```python
from build123d import *

# Parameters (mm, degrees)
SKETCH1_W                = 254
SKETCH1_H                = 508
BOSS_EXTRUDE1_DEPTH      = 203.2
FILLET1_RADIUS           = 101.6
FILLET1_LENGTH           = 254
BOSS_EXTRUDE2_DEPTH      = 25.4
BOSS_EXTRUDE2_DEPTH_BACK = 279.4
SKETCH2_R                = 12.7
CUT_EXTRUDE1_DEPTH       = 195.834
CUT_EXTRUDE1_DEPTH_BACK  = 440.182
SKETCH4_R                = 12.7


with BuildPart() as part:
    # Sketch1 → Boss-Extrude1 (new body)
    with BuildSketch(Plane.XY):
        with Locations((127, 254)):
            Rectangle(SKETCH1_W, SKETCH1_H)
    extrude(amount=BOSS_EXTRUDE1_DEPTH)

    # Fillet1: full round fillet: the end face becomes a half cylinder, R = half its width
    fillet1_face = Plane((127, 0, 101.6), x_dir=(1, 0, 0), z_dir=(0, -1, 0))  # on the end face: x along it, z out of the body
    fillet1_slab = fillet1_face.offset(-FILLET1_RADIUS / 2) * Box(FILLET1_LENGTH, 2 * FILLET1_RADIUS, FILLET1_RADIUS, mode=Mode.PRIVATE)  # the body's end, R deep
    fillet1_round = Plane((127, 101.6, 101.6), x_dir=(0, -1, 0), z_dir=(1, 0, 0)) * Cylinder(FILLET1_RADIUS, FILLET1_LENGTH, mode=Mode.PRIVATE)  # its axis R under the face
    add(fillet1_slab - fillet1_round, mode=Mode.SUBTRACT)

    # Sketch2 → Boss-Extrude2 (add, two sides: drawn at the far end of the back side and taken through both)
    with BuildSketch(Plane(origin=(254, 0, 0), x_dir=(0, 0, -1), z_dir=(1, 0, 0)).offset(-BOSS_EXTRUDE2_DEPTH_BACK)):
        with Locations((-101.6, 25.4)):
            Circle(SKETCH2_R)
    extrude(amount=BOSS_EXTRUDE2_DEPTH + BOSS_EXTRUDE2_DEPTH_BACK)

    # Sketch4 → Cut-Extrude1 (cut, two sides: drawn at the far end of the back side and taken through both)
    with BuildSketch(Plane(origin=(254, 0, 0), x_dir=(0, 0, -1), z_dir=(1, 0, 0)).offset(-CUT_EXTRUDE1_DEPTH_BACK)):
        with Locations(Location((-101.6, 482.6, 0), (0, 0, 180))):
            Circle(SKETCH4_R)
    extrude(amount=CUT_EXTRUDE1_DEPTH + CUT_EXTRUDE1_DEPTH_BACK, mode=Mode.SUBTRACT)


solid = part.part
```
Verification items for the finished model (mm, model axes). A direction names the side the tool comes from. Give positions to 0.01 mm unless a question says otherwise; leave off trailing zeros. Order: outer loops, then holes, each group sorted by start corner. A loop starts at its lowest first (then second) coordinate and runs counter-clockwise, first axis right, second up. Notation, with made-up numbers: M 43,26.5 L 93,26.5 A31 ccw 93,56.5 Z; hole C 27.5,10 d10. An arc over 180 degrees is marked long. Answer in a Markdown table with one row per item. Add a question column.
Item 1: Section check B-B, the plane z = 101.6. Enter the section's corners in (x, y), and give its area (3 significant figures).
Item 2: Scan lines: probe 1 along Z at (x, y) = (181, 482); probe 2 along X at (y, z) = (335.5, 27); probe 3 along Y at (x, z) = (164.5, 101.6). Record each from-to range of solid material in increasing order. Write a range as from..to.
Item 3: Section check A-A, the plane y = 482.6. Enter the section's corners in (x, z), and give its area (3 significant figures).
Item 4: Gauge pin test, flat ends, axial feed: pin 1 (12 mm diameter, centred on y = 211, z = 75, fed in from -X); pin 2 (5 mm diameter, centred on y = 252.5, z = 121.5, fed in from +X); pin 3 (4 mm diameter, centred on x = 227, z = 167, fed in from -Y); pin 4 (20.5 mm diameter, centred on y = 482.6, z = 101.6, fed in from -X). Record the tip position at first contact, or that the pin passes through.
Item 5: Tool access check on faces 1 (the flat face through (125, 508, 100)), 2 (the cylindrical face through (-12.878, 29.215, 89.486)), 3 (the cylindrical face through (266.522, 29.215, 89.486)). Record the directions out of +Z, -Z, +X, -X, +Y, -Y that give a thin tool (end or side, any length) a straight path to the whole face; none if there is none.
Item 6: Section check D-D, the plane y = 25.4. Enter the section's corners in (x, z).
Item 7: Mould release check, pull along Z, two halves, no side actions. Record for faces 4 (the cylindrical face through (128.778, 0.025, 103.834)), 5 (the flat face through (254, 250, 100)), 6 (the flat face through (125, 308, 0)), 7 (the cylindrical face through (125.22, 495, 98.85)): released by +Z, released by -Z, zero draft, split by the parting line, or undercut.
Item 8: Section check C-C, the plane x = 9. Enter the section's corners in (y, z).
Filled sheet:
| question | item | result |
|---|---|---|
| 1 | outline | M -25.4,12.7 L 0,12.7 L 0,0 L 254,0 L 254,12.7 L 279.4,12.7 L 279.4,38.1 L 254,38.1 L 254,469.9 L 0,469.9 L 0,38.1 L -25.4,38.1 Z; M 0,495.3 L 254,495.3 L 254,508 L 0,508 Z |
| 1 | area | 124,000 mm^2 |
| 2 | probe 1 | z = 0..88.91, 114.29..203.2 |
| 2 | probe 2 | x = 0..254 |
| 2 | probe 3 | y = 0..469.9, 495.3..508 |
| 3 | outline | M 0,0 L 254,0 L 254,88.9 L 0,88.9 Z; M 0,114.3 L 254,114.3 L 254,203.2 L 0,203.2 Z |
| 3 | area | 45,200 mm^2 |
| 4 | pin 1 | stops at x = 0 |
| 4 | pin 2 | stops at x = 254 |
| 4 | pin 3 | stops at y = 22.21 |
| 4 | pin 4 | passes through |
| 5 | face 1 | +Z, -Z, +X, -X, +Y |
| 5 | face 2 | -X |
| 5 | face 3 | +X |
| 6 | outline | M -25.4,88.9 L 0,88.9 L 0,34.4 L 254,34.4 L 254,88.9 L 279.4,88.9 L 279.4,114.3 L 254,114.3 L 254,168.8 L 0,168.8 L 0,114.3 L -25.4,114.3 Z |
| 7 | face 4 | split by the parting line |
| 7 | face 5 | zero draft |
| 7 | face 6 | released by -Z |
| 7 | face 7 | undercut |
| 8 | outline | M 101.6,0 L 508,0 L 508,203.2 L 101.6,203.2 A101.6 ccw Z; hole C 482.6,101.6 d25.4 |
